For this review, take the finished solid that the model builds, in its own axes (mm). Face numbers are marked on the shaded views. A direction names the side the tool comes from. Coordinates: 2 decimals unless noted, no trailing zeros. Loops run counter-clockwise (first coordinate to the right, second up) from the corner with the lowest first, then second, coordinate; pieces in that order, holes last. Notation, with made-up numbers: (57.5, 79.25) -> (64.5, 79.25) arc R18 ccw to (64.5, 83.25) -> close; hole circle Ø6 at (66.25, 80.5). An arc over 180 degrees is marked (long way). One line per item, written item: value.
from build123d import *

# Parameters (mm, degrees)
SKETCH1_R                = 8.75
BOSS_EXTRUDE1_DEPTH      = 2
THREADEDHOLES_REACH      = 26.678
THREADEDHOLES_END_RADIUS = 8.75
SKETCH2_R                = 1.25


with BuildPart() as part:
    # Sketch1 → Boss-Extrude1 (new, symmetric)
    with BuildSketch(Plane.XY):
        with BuildLine():
            Line((8.75, 11), (-8.75, 11))
            Line((-8.75, 11), (-10.718127175, 2.47421702))
            ThreePointArc((-10.718127175, 2.47421702), (0, -11), (10.718127175, 2.47421702))
            Line((10.718127175, 2.47421702), (8.75, 11))
        make_face()
        Circle(SKETCH1_R, mode=Mode.SUBTRACT)
    extrude(amount=BOSS_EXTRUDE1_DEPTH, both=True)

    # ThreadedHoles: up to this cylinder (the profile starts outside it)
    threadedholes_end = Plane(origin=(0, 0, 0), z_dir=(0, 0, -1)) * Cylinder(THREADEDHOLES_END_RADIUS, 71.856, mode=Mode.PRIVATE)
    # Sketch2 → ThreadedHoles (cut, up to the surface)
    with BuildSketch(Plane(origin=(0, 11, 0), x_dir=(1, 0, 0), z_dir=(0, 1, 0)), mode=Mode.PRIVATE) as threadedholes_sk1:
        with Locations(Location((-5, 0, 0), (0, 0, 180))):
            Circle(SKETCH2_R)
    threadedholes_tool1 = extrude(threadedholes_sk1.sketch, amount=-THREADEDHOLES_REACH, mode=Mode.PRIVATE) - threadedholes_end
    add(threadedholes_tool1.solids().sort_by_distance((-5, 11, 0))[0], mode=Mode.SUBTRACT)
    # Sketch2 → ThreadedHoles (cut, up to the surface)
    with BuildSketch(Plane(origin=(0, 11, 0), x_dir=(1, 0, 0), z_dir=(0, 1, 0)), mode=Mode.PRIVATE) as threadedholes_sk2:
        with Locations(Location((5, 0, 0), (0, 0, 180))):
            Circle(SKETCH2_R)
    threadedholes_tool2 = extrude(threadedholes_sk2.sketch, amount=-THREADEDHOLES_REACH, mode=Mode.PRIVATE) - threadedholes_end
    add(threadedholes_tool2.solids().sort_by_distance((5, 11, 0))[0], mode=Mode.SUBTRACT)


solid = part.part
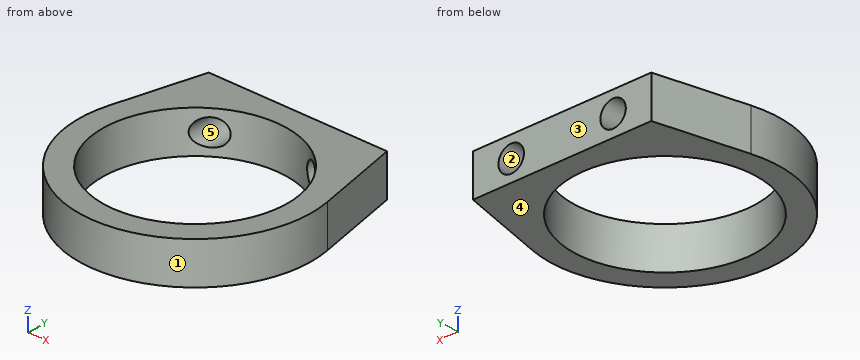
1. Take a section at B-B, the plane y = -2.5. Give the boundary of the cut face in (x, z), and give its area (3 significant figures).
Return value:
outline: (-10.71, -2) -> (-8.39, -2) -> (-8.39, 2) -> (-10.71, 2) -> close; (8.39, -2) -> (10.71, -2) -> (10.71, 2) -> (8.39, 2) -> close
area: 18.6 mm2
2. Insertion check: pin 1 Ø1 at (y, z) = (-2.5, -1) entering from -X; pin 2 Ø2 at (x, z) = (5, 0) entering from -Y; pin 3 Ø2 at (x, z) = (7.5, 1) entering from -Y. Each pin has a flat end and moves straight along its axis. Give the tip position at first contact, or say it passes through.
Return value:
pin 1: stops at x = -10.82
pin 2: stops at y = -10.25
pin 3: stops at y = -8.87
3. Take a section at A-A, the plane x = 0. Give the boundary of the cut face in (y, z), and give its area (3 significant figures).
Return value:
outline: (-11, -2) -> (-8.75, -2) -> (-8.75, 2) -> (-11, 2) -> close; (8.75, -2) -> (11, -2) -> (11, 2) -> (8.75, 2) -> close
area: 18.0 mm2
4. For the marked faces 1 and 2, list the 3-axis set-ups (+Z, -Z, +X, -X, +Y, -Y) from which the entire face can be reached by the end or side of a thin tool; tool diameter is ignored.
Return value:
face 1: +Z, -Z
face 2: +Y
5. The part is to be moulded in two halves that separate along Z. For the marked faces 3, 4 and 5, say which applies: pulls with the +Z half, pulls with the -Z half, needs draft (parallel to the pull), parting line crosses it, or undercut.
Return value:
face 3: needs draft
face 4: pulls with the -Z half
face 5: undercut
6. Take a section at D-D, the plane x = -5. Give the boundary of the cut face in (y, z), and give its area (3 significant figures).
Return value:
outline: (-9.8, -2) -> (-7.18, -2) -> (-7.18, 2) -> (-9.8, 2) -> close; (7.18, -2) -> (11, -2) -> (11, -1.25) -> (7.18, -1.25) -> close; (7.18, 1.25) -> (11, 1.25) -> (11, 2) -> (7.18, 2) -> close
area: 16.2 mm2
7. To check wall thickness, follow probe 1 along Y at (x, z) = (0, 1.05); probe 2 along X at (y, z) = (9.4, 0); probe 3 along Z at (x, y) = (5, 7.45). State the ranges of each line that lie inside material, in increasing order. Write a range as from..to.
Return value:
probe 1: y = -11..-8.75, 8.75..11
probe 2: x = -9.12..-6.25, -3.75..3.75, 6.25..9.12
probe 3: z = -2..-1.25, 1.25..2
8. Take a section at C-C, the plane z = 0. Give the boundary of the cut face in (x, y), and give its area (3 significant figures).
Return value:
outline: (-10.72, 2.47) arc R11 ccw (long way) to (10.72, 2.47) -> (8.75, 11) -> (6.25, 11) -> (6.25, 6.12) arc R8.75 cw (long way) to (-6.25, 6.12) -> (-6.25, 11) -> (-8.75, 11) -> close; (-3.75, 7.91) arc R8.75 cw to (3.75, 7.91) -> (3.75, 11) -> (-3.75, 11) -> close
area: 150 mm2
